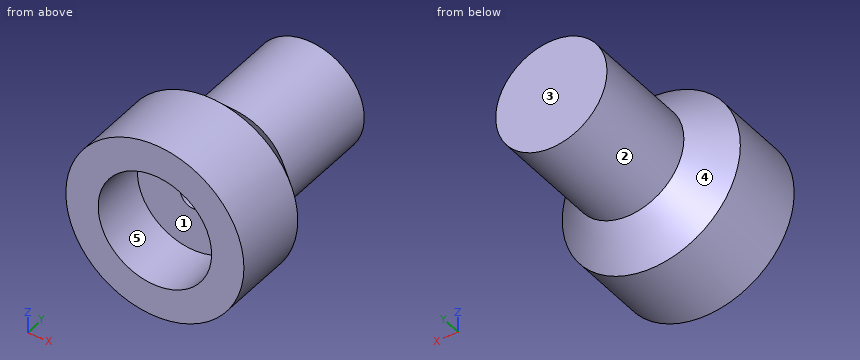
```python
from build123d import *

# Parameters (mm, degrees)
CHAMFER_1_SIZE       = 3
SKETCH_4_R           = 5.1
CUT_EXTRUDE_1_DEPTH  = 5.1
HOLE_WIZARD_M3_D     = 2.5
HOLE_WIZARD_M3_DEPTH = 10
HOLE_WIZARD_M3_TIP   = 0.751075774


with BuildPart() as part:
    # Эскиз1 → Revolve 482 (revolve)
    with BuildSketch(Plane.XY):
        Polygon((0, 10), (-5, 10), (-5, 0), (-8, 0), (-8, -10), (0, -10), align=None)
    revolve(axis=Axis((0, 10, 0), (0, -1, 0)))

    # Фаска1
    chamfer_1_edges = [part.edges().sort_by_distance(p)[0] for p in [
        (8, 0, 0),
    ]]
    chamfer(chamfer_1_edges, length=CHAMFER_1_SIZE - 0.0001)  # a hair under: the kernel refuses the full size

    # Эскиз4 → Вырез-Вытянуть1 (cut)
    with BuildSketch(Plane.XZ.offset(10)):
        Circle(SKETCH_4_R)
    extrude(amount=-CUT_EXTRUDE_1_DEPTH, mode=Mode.SUBTRACT)

    # Крепление магнита M3
    with Locations(Plane(origin=(0, -4.9, 0), x_dir=(-1, 0, 0), z_dir=(0, -1, 0))):
        with Locations((0, 0)):
            Hole(HOLE_WIZARD_M3_D / 2, depth=HOLE_WIZARD_M3_DEPTH)
            with Locations((0, 0, -(HOLE_WIZARD_M3_DEPTH + HOLE_WIZARD_M3_TIP / 2))):  # 118° drill point
                Cone(0, HOLE_WIZARD_M3_D / 2, HOLE_WIZARD_M3_TIP, mode=Mode.SUBTRACT)


solid = part.part
```
Can you work these out from the model? Positions are in its coordinate system, mm. Face numbers are marked on the shaded views. A direction names the side the tool comes from. Round coordinates to 2 decimals unless told otherwise and drop trailing zeros. Loops run counter-clockwise (first coordinate to the right, second up) from the corner with the lowest first, then second, coordinate; pieces in that order, holes last. Notation, with made-up numbers: M 80,-25 L 107,-25 A22 cw 107,-1 Z; hole C 55.5,23.25 d11. An arc over 180 degrees is marked long. Answer in a Markdown table with one row per item.
1. If we section it at B-B, the plane y = 1.25: Please give me the cut outline in (x, z), plus the area to 3 significant figures.
Established:
| item | result |
|---|---|
| outline | C 0,0 d10; hole C 0,0 d2.5 |
| area | 73.6 mm² |
2. If we section it at A-A, the plane y = -5.5: Please give me the cut outline in (x, z).
Established:
| item | result |
|---|---|
| outline | C 0,0 d16; hole C 0,0 d10.2 |
3. On a 3-axis mill with a long thin cutter (end or side, diameter ignored), from which of +Z, -Z, +X, -X, +Y, -Y can I reach the whole of each face in a straight line? I mean the marked faces 4 and 5. Say none if no direction works.
Established:
| item | result |
|---|---|
| face 4 | +Y |
| face 5 | -Y |
4. Please list where these lines run through material, in increasing order: line 1 (Z direction, x = 0, y = 0.25); line 2 (X direction, y = -3.25, z = 0.25); line 3 (Z direction, x = 0, y = -0.75). Write a range as from..to.
Established:
| item | result |
|---|---|
| line 1 | -5..-1.25, 1.25..5 |
| line 2 | -8..-1.22, 1.22..8 |
| line 3 | -5.75..-1.25, 1.25..5.75 |
5. I'm going to push flat-ended pins straight in: pin 1 Ø8 at (y, z) = (4.5, -3.5) entering from -X; pin 2 Ø4 at (y, z) = (0, -4.5) entering from -X; pin 3 Ø5 at (x, z) = (-1, 1.5) entering from -Y. Where does each tip first touch, or does it pass through?
Established:
| item | result |
|---|---|
| pin 1 | x = -5 |
| pin 2 | x = -5.75 |
| pin 3 | y = -4.9 |
6. Thinking about a two-plate mould opening in Z: for the marked faces 1, 2 and 3, which applies, pulls with the +Z half, pulls with the -Z half, needs draft (parallel to the pull), parting line crosses it, or undercut?
Established:
| item | result |
|---|---|
| face 1 | undercut |
| face 2 | parting line crosses it |
| face 3 | needs draft |
